from build123d import *

# Parameters (mm, degrees)
SKETCH1_R               = 2.9
BOSS_EXTRUDE1_DEPTH     = 15
FILLET2_R               = 1
SKETCH2_W               = 5.8
SKETCH2_H               = 5
SKETCH2_R               = 1
CUT_EXTRUDE1_DEPTH      = 0.75
CUT_EXTRUDE2_DEPTH      = 16.550562691
CUT_EXTRUDE2_DEPTH_BACK = 16.550562691
SKETCH2_3_R             = 1
FILLET4_R               = 0.2


with BuildPart() as part:
    # Sketch1 → Boss-Extrude1 (new body)
    with BuildSketch(Plane.XY):
        Circle(SKETCH1_R)
    extrude(amount=BOSS_EXTRUDE1_DEPTH)

    # Fillet2
    fillet2_edges = [part.edges().sort_by_distance(p)[0] for p in [
        (-2.9, 0, 0),
    ]]
    fillet(fillet2_edges, radius=FILLET2_R)

    # Sketch2 → Cut-Extrude1 (cut, symmetric)
    # profile 1 of 2: a face of its own
    with BuildSketch(Plane(origin=(0, 0, 0), x_dir=(1, 0, 0), z_dir=(0, 1, 0))):
        with Locations((0, -12.5)):
            Rectangle(SKETCH2_W, SKETCH2_H)
        with Locations((0, -12.5)):
            Circle(SKETCH2_R, mode=Mode.SUBTRACT)
    # profile 2 of 2: a face of its own
    with BuildSketch(Plane(origin=(0, 0, 0), x_dir=(1, 0, 0), z_dir=(0, 1, 0))):
        with Locations((0, -12.5)):
            Circle(SKETCH2_R)
    extrude(amount=CUT_EXTRUDE1_DEPTH, both=True, mode=Mode.SUBTRACT)

    # Sketch2_3 → Cut-Extrude2 (cut, two sides: drawn at the far end of the back side and taken through both)
    with BuildSketch(Plane(origin=(0, 0, 0), x_dir=(1, 0, 0), z_dir=(0, 1, 0)).offset(-CUT_EXTRUDE2_DEPTH_BACK)):
        with Locations(Location((0, -12.5, 0), (0, 0, 270))):
            Circle(SKETCH2_3_R)
    extrude(amount=CUT_EXTRUDE2_DEPTH + CUT_EXTRUDE2_DEPTH_BACK, mode=Mode.SUBTRACT)

    # Fillet4
    fillet4_edges = [part.edges().sort_by_distance(p)[0] for p in [
        (0, 0.75, 15),
        (0, -0.75, 15),
        (0, 2.9, 15),
        (0, -2.9, 15),
    ]]
    fillet(fillet4_edges, radius=FILLET4_R)


solid = part.part
Can you work these out from the model? Positions are in its coordinate system, mm. A direction names the side the tool comes from. Round coordinates to 2 decimals unless told otherwise and drop trailing zeros. Order: outer loops, then holes, each group sorted by start corner. A loop starts at its lowest first (then second) coordinate and runs counter-clockwise, first axis right, second up. Notation, with made-up numbers: (17, 35) -> (26, 35) arc R29 cw to (26, 59) -> close; hole circle Ø11 at (58, 14.25). An arc over 180 degrees is marked (long way). Write each question's results on one line, items separated by ' | '. Start each with the question number.
Item 1: If we section it at A-A, the plane x = 0: Write out the boundary of the cut face in (y, z), then the cut area to 3 significant figures.
Item 2: If we section it at D-D, the plane z = 1.5: Write out the boundary of the cut face in (x, y), then the cut area to 3 significant figures.
Item 3: Please list where these lines run through material, in increasing order: L1, parallel to Z at x = 0, y = -1.3; L2, parallel to X at y = 1.05, z = 5; L3, parallel to Z at x = 1.5, y = 0.7.
Item 4: Which directions (+Z, -Z, +X, -X, +Y, -Y) give clear straight access to the entire face, cutting with the end or side of a thin tool? Please do faces 1 (the cylindrical face through (2.766, 0.871, 7.803)), 2 (the flat face through (0, -0.75, 11)).
Item 5: Will these pins go through, and if not, where does the flat tip stop? pin 1 (1.5 mm diameter, centred on y = 1, z = 8, fed in from -X); pin 2 (1 mm diameter, centred on y = 1, z = 11, fed in from +X).
Item 6: If we section it at C-C, the plane y = 0: Write out the boundary of the cut face in (x, z), then the cut area to 3 significant figures.
Item 7: Thinking about a two-plate mould opening in Z: for faces 3 (the cylindrical face through (0, -1.8, 11.5)), 4 (the flat face through (0, 0, 0)), 5 (the flat face through (0, 0, 10)), which applies, +Z half, -Z half, draft (parallel to the pull), parting line (faces both ways), or undercut?
Item 8: If we section it at B-B, the plane z = 11: Write out the boundary of the cut face in (x, y).
Results:
1) outline: (-2.9, 1) arc R1 ccw to (-1.9, 0) -> (1.9, 0) arc R1 ccw to (2.9, 1) -> (2.9, 11.5) -> (0.75, 11.5) -> (0.75, 10) -> (-0.75, 10) -> (-0.75, 11.5) -> (-2.9, 11.5) -> close; (-2.9, 13.5) -> (-0.75, 13.5) -> (-0.75, 14.8) arc R0.2 ccw to (-0.95, 15) -> (-2.7, 15) arc R0.2 ccw to (-2.9, 14.8) -> close; (0.75, 13.5) -> (2.9, 13.5) -> (2.9, 14.8) arc R0.2 ccw to (2.7, 15) -> (0.95, 15) arc R0.2 ccw to (0.75, 14.8) -> close | area: 70.4 mm2
2) outline: circle Ø5.8 at (0, 0) | area: 26.4 mm2
3) L1: z = 0 to 11.5, 13.5 to 15 | L2: x = -2.7 to 2.7 | L3: z = 0 to 10
4) face 1: +Z, -Z | face 2: +Z, +X, -X
5) pin 1: stops at x = -2.89 | pin 2: stops at x = 2.8
6) outline: (-2.9, 1) arc R1 ccw to (-1.9, 0) -> (1.9, 0) arc R1 ccw to (2.9, 1) -> (2.9, 10) -> (-2.9, 10) -> close | area: 57.6 mm2
7) face 3: undercut | face 4: -Z half | face 5: +Z half
8) outline: (-2.8, -0.75) arc R2.9 ccw to (2.8, -0.75) -> close; (-2.8, 0.75) -> (2.8, 0.75) arc R2.9 ccw to start
